Part model, mm, in its own coordinate system. A direction names the side the tool comes from. Round coordinates to 2 decimals unless told otherwise and drop trailing zeros. Loops run counter-clockwise (first coordinate to the right, second up) from the corner with the lowest first, then second, coordinate; pieces in that order, holes last. Notation, with made-up numbers: M 70,87 L 110,87 A6 cw 110,92 Z; hole C -11,43 d2. An arc over 180 degrees is marked long. Answer as CSV lines item,"result". Start each with the question number.
Item 1: Which spindle directions (+Z, -Z, +X, -X, +Y, -Y) get a long thin tool onto all of the face, cutting with end or side? Do faces 1 (the flat face through (238, -23, 35)), 2 (the cylindrical face through (249.027, -8.857, -8.753)), 3 (the cylindrical face through (254.66, 35.425, 15.168)). Say none if no direction does.
Item 2: Band-saw the part on A-A (z = 27). Give the cut face in (x, y).
Item 3: Drop flat-ended pins along their axis: pin 1 Ø1.1 at (x, z) = (244.5, 22.5) entering from +Y; pin 2 Ø1 at (x, y) = (246, -23.5) entering from +Z; pin 3 Ø0.5 at (y, z) = (-9.5, 15) entering from +X; pin 4 Ø6.5 at (x, y) = (246.5, -7.5) entering from +Z. Give the stop position or say it passes through.
Item 4: Wall check: line 1 (Y direction, x = 249.15, z = 12); line 2 (Z direction, x = 245.35, y = 9); line 3 (Z direction, x = 248.75, y = 9). Give the ranges that are in metal, low to high.
Item 5: Band-saw the part on B-B (y = -32). Give the cut face in (x, z).
Item 6: Band-saw the part on C-C (z = 12). Count the separate pieces of the cut face and the enclosed holes in it, and give its area (3 significant figures).
Item 7: Mould opens along Y. For faces 4 (the flat face through (253, 18.5, 8)), 5 (the flat face through (248, -10.4, -13.4)), 6 (the flat face through (252.82, 0.59, 21.96)) say: pulls with the +Y half, pulls with the -Y half, needs draft (parallel to the pull), parting line crosses it, or undercut.
```python
from build123d import *

# Parameters (mm, degrees)
SKETCH_1_W          = 52.8
SKETCH_1_H          = 84
EXTRUDE_1_DEPTH     = 6
SKETCH_2_R          = 1.5
CUT_EXTRUDE_1_DEPTH = 8
SKETCH_3_W          = 60
SKETCH_3_H          = 46
CUT_EXTRUDE_2_DEPTH = 50
EXTRUDE_2_DEPTH     = 40
EXTRUDE_3_DEPTH     = 6
EXTRUDE_4_DEPTH     = 6
SKETCH_7_R          = 1.6
CUT_EXTRUDE_3_DEPTH = 70
SKETCH_8_R          = 3.25
CUT_EXTRUDE_4_DEPTH = 12
SKETCH_9_R          = 4
CUT_EXTRUDE_5_DEPTH = 23.5


with BuildPart() as part:
    # 草图1 → 凸台-拉伸1 (new body)
    with BuildSketch(Plane(origin=(159.175409567, 0, 133.564027461), x_dir=(0.6427876096867067, 0, -0.7660444431188377), z_dir=(0.7660444431188378, 0, 0.6427876096867067))):
        with Locations((140.187338197, 0)):
            Rectangle(SKETCH_1_W, SKETCH_1_H)
    extrude(amount=-EXTRUDE_1_DEPTH)

    # 草图2 → 切除-拉伸1 (cut)
    with BuildSketch(Plane(origin=(159.175409567, 0, 133.564027461), x_dir=(0.6427876096867067, 0, -0.7660444431188377), z_dir=(0.7660444431188378, 0, 0.6427876096867067))):
        with Locations((117.287338197, -36)):
            Circle(SKETCH_2_R)
        with Locations((117.287338197, 36)):
            Circle(SKETCH_2_R)
        with Locations((150.687338197, 36)):
            Circle(SKETCH_2_R)
        with Locations((128.687338197, 36)):
            Circle(SKETCH_2_R)
        with Locations((128.687338197, -36)):
            Circle(SKETCH_2_R)
        with Locations((162.087338197, 36)):
            Circle(SKETCH_2_R)
        with Locations((162.087338197, -36)):
            Circle(SKETCH_2_R)
        with Locations((150.687338197, -36)):
            Circle(SKETCH_2_R)
    extrude(amount=-CUT_EXTRUDE_1_DEPTH, mode=Mode.SUBTRACT)

    # 草图3 → 切除-拉伸2 (cut)
    with BuildSketch(Plane.XY.offset(25)):
        with Locations((250, 0)):
            Rectangle(SKETCH_3_W, SKETCH_3_H)
    extrude(amount=CUT_EXTRUDE_2_DEPTH, mode=Mode.SUBTRACT)

    # 草图4 → 凸台-拉伸2 (add)
    with BuildSketch(Plane(origin=(0, 20, 0), x_dir=(-1, 0, 0), z_dir=(0, -1, 0))):
        with BuildLine():
            Line((-249.1237949, 22), (-243.086632908, 22))
            add(Edge.make_bspline(
                [(-243.086632908, 22), (-243.481254737, 18.531426174), (-243.784948463, 14.933770973), (-243.993041019, 11.223078881), (-244.1, 7.416444076), (-244.1, 3.53121788)],
                knots=[0.778865295, 0.778865295, 0.778865295, 0.778865295, 0.778865295, 0.778865295, 1, 1, 1, 1, 1, 1], degree=5))
            add(Edge.make_bspline(
                [(-244.1, 3.53121788), (-244.1, -1.069863619), (-243.955995612, -5.56513348), (-243.676385618, -9.929661799), (-243.268946043, -14.139045721), (-242.741071446, -18.169549128), (-242.097814731, -22)],
                knots=[0, 0, 0, 0, 0, 0, 0, 0.314254692, 0.314254692, 0.314254692, 0.314254692, 0.314254692, 0.314254692, 0.314254692], degree=6))
            Line((-242.097814731, -22), (-248.177885229, -22))
            add(Edge.make_bspline(
                [(-248.177885229, -22), (-248.800145217, -18.111595668), (-249.307087627, -14.054845034), (-249.696626763, -9.84368942), (-249.96306742, -5.496084567), (-250.1, -1.031127344), (-250.1, 3.53121788)],
                knots=[0.698640687, 0.698640687, 0.698640687, 0.698640687, 0.698640687, 0.698640687, 0.698640687, 1, 1, 1, 1, 1, 1, 1], degree=6))
            add(Edge.make_bspline(
                [(-250.1, 3.53121788), (-250.1, 7.398092065), (-249.997534101, 11.192091342), (-249.797793696, 14.899179655), (-249.505456591, 18.505771646), (-249.1237949, 22)],
                knots=[0, 0, 0, 0, 0, 0, 0.212850791, 0.212850791, 0.212850791, 0.212850791, 0.212850791, 0.212850791], degree=5))
        make_face()
    extrude(amount=EXTRUDE_2_DEPTH)

    # 草图5 → 凸台-拉伸3 (add)
    with BuildSketch(Plane(origin=(0, -18.5, 0), x_dir=(-1, 0, 0), z_dir=(0, -1, 0))):
        Polygon((-246, -4), (-266, -4), (-250, -23), (-244, -23), align=None)
    extrude(amount=-EXTRUDE_3_DEPTH)

    # 草图6 → 凸台-拉伸4 (add)
    with BuildSketch(Plane(origin=(0, 12.5, 0), x_dir=(-1, 0, 0), z_dir=(0, -1, 0))):
        Polygon((-246, -4), (-266, -4), (-250, -23), (-244, -23), align=None)
    extrude(amount=-EXTRUDE_4_DEPTH)

    # 草图7 → 切除-拉伸3 (cut)
    with BuildSketch(Plane(origin=(285, 0, 0), x_dir=(0, 0, -1), z_dir=(1, 0, 0))):
        with Locations((12, -9)):
            Circle(SKETCH_7_R)
        with Locations((-12, -9)):
            Circle(SKETCH_7_R)
        with Locations((12, 9)):
            Circle(SKETCH_7_R)
        with Locations((-12, 9)):
            Circle(SKETCH_7_R)
    extrude(amount=-CUT_EXTRUDE_3_DEPTH, mode=Mode.SUBTRACT)

    # 草图8 → 切除-拉伸4 (cut)
    with BuildSketch(Plane(origin=(260, 0, 0), x_dir=(0, 0, -1), z_dir=(1, 0, 0))):
        with Locations((12, -9)):
            Circle(SKETCH_8_R)
        with Locations((-12, -9)):
            Circle(SKETCH_8_R)
        with Locations((12, 9)):
            Circle(SKETCH_8_R)
        with Locations((-12, 9)):
            Circle(SKETCH_8_R)
    extrude(amount=-CUT_EXTRUDE_4_DEPTH, mode=Mode.SUBTRACT)

    # 草图9 → 切除-拉伸5 (cut)
    with BuildSketch(Plane(origin=(275, 0, 0), x_dir=(0, 0, -1), z_dir=(1, 0, 0))):
        with Locations((-12, -9)):
            Circle(SKETCH_9_R)
        with Locations((-12, 9)):
            Circle(SKETCH_9_R)
    extrude(amount=-CUT_EXTRUDE_5_DEPTH, mode=Mode.SUBTRACT)


solid = part.part
```
Answer block:
1,face 1,"+Z, +X, -X"
1,face 2,"+X"
1,face 3,"none"
2,outline,"M 240.76,-42 L 248.59,-42 L 248.59,-23 L 240.76,-23 Z; M 240.76,23 L 248.59,23 L 248.59,42 L 240.76,42 Z"
3,pin 1,"stops at y = 42"
3,pin 2,"stops at z = 30.69"
3,pin 3,"stops at x = 251.5"
3,pin 4,"stops at z = 25"
4,line 1,"y = -20 to -12.25, -5.75 to 5.75, 12.25 to 20"
4,line 2,"z = -22 to -13.6, -10.4 to 10.4, 13.6 to 25"
4,line 3,"z = -22 to -15.25, -8.75 to 8.75, 15.25 to 25"
5,outline,"M 227.72,42.54 L 261.66,2.09 L 266.26,5.95 L 232.32,46.4 Z"
6,separate pieces,"4"
6,enclosed holes,"0"
6,area,"771 mm^2"
7,face 4,"pulls with the +Y half"
7,face 5,"undercut"
7,face 6,"needs draft"
